```python
from build123d import *

# Parameters (mm, degrees)
F2_W     = 15
F2_H     = 15
F3_DEPTH = 1


with BuildPart() as f1:
    # F0 (on Front) → F1 (revolve)
    with BuildSketch(Plane.XZ):
        Polygon((-5.123077, 1.89), (-5.123077, 0.5), (20.616923, 0.5), (20.616923, 1.42), (20.246923, 1.89), (8.966923, 1.89), (7.836923, 2.31), (7.286923, 2.31), (6.576923, 1.89), (2.416923, 1.89), (2.021923, 4.26), (1.081923, 4.26), (0.686923, 1.89), (0, 1.89), align=None)
    revolve(axis=Axis((9.142162, 0, 0), (1, 0, 0)))

    # F2 (on face) → F3 (join)
    with BuildSketch(Plane(origin=(-5.123077, 0, 0), x_dir=(0, -1, 0), z_dir=(-1, 0, 0))):
        Rectangle(F2_W, F2_H)
    extrude(amount=F3_DEPTH)


solid = f1.part
```
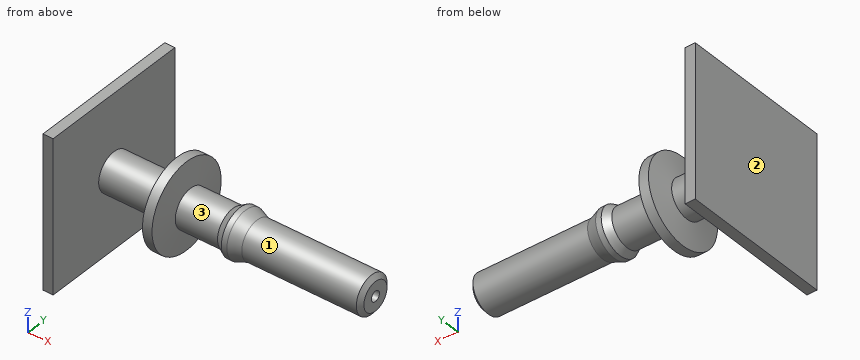
The listing builds one solid part. Answer for the finished solid, in the listing's coordinates (mm). Face numbers are marked on the shaded views. Round coordinates to 2 decimals unless told otherwise and drop trailing zeros. Loops run counter-clockwise (first coordinate to the right, second up) from the corner with the lowest first, then second, coordinate; pieces in that order, holes last. Notation, with made-up numbers: (-27, -1) - (2, -1) arc R25 cw to (2, 29) - close; hole circle Ø8 at (66.5, 87.5). An arc over 180 degrees is marked (long way). Return JSON: item names as keys, results as strings. Group by question number.
1. Consider probe 1 along Z at (x, y) = (5, 0); probe 2 along X at (y, z) = (-4.5, -1.5). Determine where each line is inside the solid, lowest interval first.
2. The mould has two halves that part along X. Classify the marked faces 1, 2 and 3: pulls with the +X half, pulls with the -X half, needs draft (parallel to the pull), parting line crosses it, or undercut.
3. The part is cut by section D-D on y = 5. Determine the outline of the cut face in (x, z), then the cut area to 3 significant figures.
4. Each of these flat-tipped pins is pushed along its axis until it touches: P1, Ø6, axis at x = -3, z = 2, coming from the +Y side; P2, Ø6, axis at x = 0, y = 1.5, coming from the +Z side; P3, Ø8, axis at x = 14, z = -2, coming from the +Y side; P4, Ø6, axis at x = 3, z = 3, coming from the -Y side. Where does it stop, or does it pass through?
5. The part is cut by section C-C on x = 19. Determine the outline of the cut face in (y, z).
Resolved:
{
 "1": {"probe 1": "z = -1.89 to -0.5, 0.5 to 1.89", "probe 2": "x = -6.12 to -5.12"},
 "2": {"face 1": "needs draft", "face 2": "pulls with the -X half", "face 3": "undercut"},
 "3": {"outline": "(-6.12, -7.5) - (-5.12, -7.5) - (-5.12, 7.5) - (-6.12, 7.5) - close", "area": "15.0 mm²"},
 "4": {"P1": "stops at y = 7.5", "P2": "stops at z = 4.26", "P3": "stops at y = 1.89", "P4": "stops at y = -4.26"},
 "5": {"outline": "circle Ø3.78 at (0, 0); hole circle Ø1 at (0, 0)"}
}
